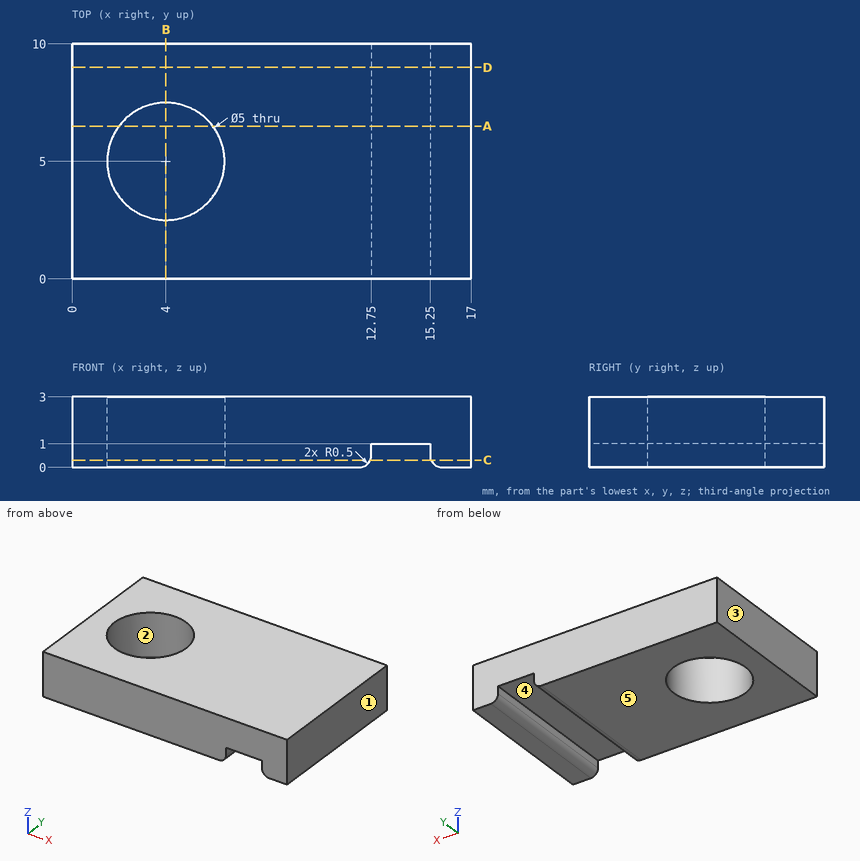
Here's the drawing with two shaded views (mm, measured from the low corner). I have some questions. A direction names the side the tool comes from. Coordinates: 2 decimals unless noted, no trailing zeros. Write each loop counter-clockwise with the first axis right and the second up, starting at its lowest first coordinate (ties: lowest second). Pieces come first, ordered by that corner, then holes. Notation, with made-up numbers: (-14, 0) -> (25, 0) arc R24 cw to (25, 33) -> close; hole circle Ø1 at (-26, 55). An arc over 180 degrees is marked (long way). Use a Markdown table: item, result. Add a question column.
(1) For the marked faces 4 and 5, which set-ups out of +Z, -Z, +X, -X, +Y, -Y let a thin tool reach every point of the face, with its end or its side?
(2) If we section it at B-B, the plane x = 4: Write out the boundary of the cut face in (y, z), and give its area (3 significant figures).
(3) We'd pull the mould along X, two halves only. Please class the marked faces 1, 2 and 3: +X half, -X half, draft (parallel to the pull), parting line (faces both ways), or undercut.
(4) If we section it at C-C, the plane z = 0.3: Write out the boundary of the cut face in (x, y), and give its area (3 significant figures).
(5) Please list where these lines run through material, in increasing order: line 1 (X direction, y = 9, z = 0.9); line 2 (Y direction, x = 4, z = 2.8); line 3 (X direction, y = 5.25, z = 2.45).
(6) If we section it at A-A, the plane y = 6.5: Write out the boundary of the cut face in (x, z), and give its area (3 significant figures).
(7) If we section it at D-D, the plane y = 9: Write out the boundary of the cut face in (x, z).
(8) I'm going to push a flat-ended pin straight in: P1, Ø0.6, axis at y = 3, z = 1, coming from the -X side. Where does the tip first touch, or does it pass through?
Outcome:
| question | item | result |
|---|---|---|
| 1 | face 4 | -Z, +Y, -Y |
| 1 | face 5 | -Z, +X, -X, +Y, -Y |
| 2 | outline | (0, 0) -> (2.5, 0) -> (2.5, 3) -> (0, 3) -> close; (7.5, 0) -> (10, 0) -> (10, 3) -> (7.5, 3) -> close |
| 2 | area | 15.0 mm^2 |
| 3 | face 1 | +X half |
| 3 | face 2 | undercut |
| 3 | face 3 | -X half |
| 4 | outline | (0, 0) -> (12.71, 0) -> (12.71, 10) -> (0, 10) -> close; (15.29, 0) -> (17, 0) -> (17, 10) -> (15.29, 10) -> close; hole circle Ø5 at (4, 5) |
| 4 | area | 125 mm^2 |
| 5 | line 1 | x = 0 to 12.75, 15.25 to 17 |
| 5 | line 2 | y = 0 to 2.5, 7.5 to 10 |
| 5 | line 3 | x = 0 to 1.51, 6.49 to 17 |
| 6 | outline | (0, 0) -> (2, 0) -> (2, 3) -> (0, 3) -> close; (6, 0) -> (12.25, 0) arc R0.5 ccw to (12.75, 0.5) -> (12.75, 1) -> (15.25, 1) -> (15.25, 0.5) arc R0.5 ccw to (15.75, 0) -> (17, 0) -> (17, 3) -> (6, 3) -> close |
| 6 | area | 36.4 mm^2 |
| 7 | outline | (0, 0) -> (12.25, 0) arc R0.5 ccw to (12.75, 0.5) -> (12.75, 1) -> (15.25, 1) -> (15.25, 0.5) arc R0.5 ccw to (15.75, 0) -> (17, 0) -> (17, 3) -> (0, 3) -> close |
| 8 | P1 | stops at x = 0 |
